Job drawing, mm, ordinate dimensions from the low corner. One solid piece. A direction names the side the tool comes from. Round coordinates to 2 decimals unless told otherwise and drop trailing zeros. Order: outer loops, then holes, each group sorted by start corner. A loop starts at its lowest first (then second) coordinate and runs counter-clockwise, first axis right, second up. Notation, with made-up numbers: (45.5, 78.5) -> (103.5, 78.5) arc R10 cw to (103.5, 96.5) -> close; hole circle Ø2 at (21.5, -22). An arc over 180 degrees is marked (long way). Return JSON: item names as keys, results as strings. Group by question number.
Q1. Which spindle directions (+Z, -Z, +X, -X, +Y, -Y) get a long thin tool onto all of the face, cutting with end or side? Do the marked faces 1, 2 and 3. Say none if no direction does.
Q2. Flat gauge pins, fed straight in: pin 1 (8 mm diameter, centred on y = 5.5, z = 30, fed in from -X); pin 2 (7.5 mm diameter, centred on x = 4.5, y = 6, fed in from +Z); pin 3 (3.5 mm diameter, centred on y = 7, z = 40, fed in from +X). Where does each tip first touch, or does it go through?
Q3. Cut at B-B (y = 11.75). Write the cut outline in (x, z).
Q4. Cut at C-C (x = 42.5). Write the cut outline in (y, z), then the cut area to 3 significant figures.
Q5. Mould opens along X. For the marked faces 4, 5 and 6 say: +X half, -X half, draft (parallel to the pull), parting line (faces both ways), or undercut.
Q6. Cut at A-A (z = 39). Write the cut outline in (x, y).
Q7. Probe line 1 along X through (y, z) = (5.5, 29); line 2 along X through (y, z) = (8, 40); line 3 along Z through (x, y) = (24, 6.5). List the from-to ranges inside material, lowest first.
Q8. Cut at D-D (z = 29). Write the cut outline in (x, y).
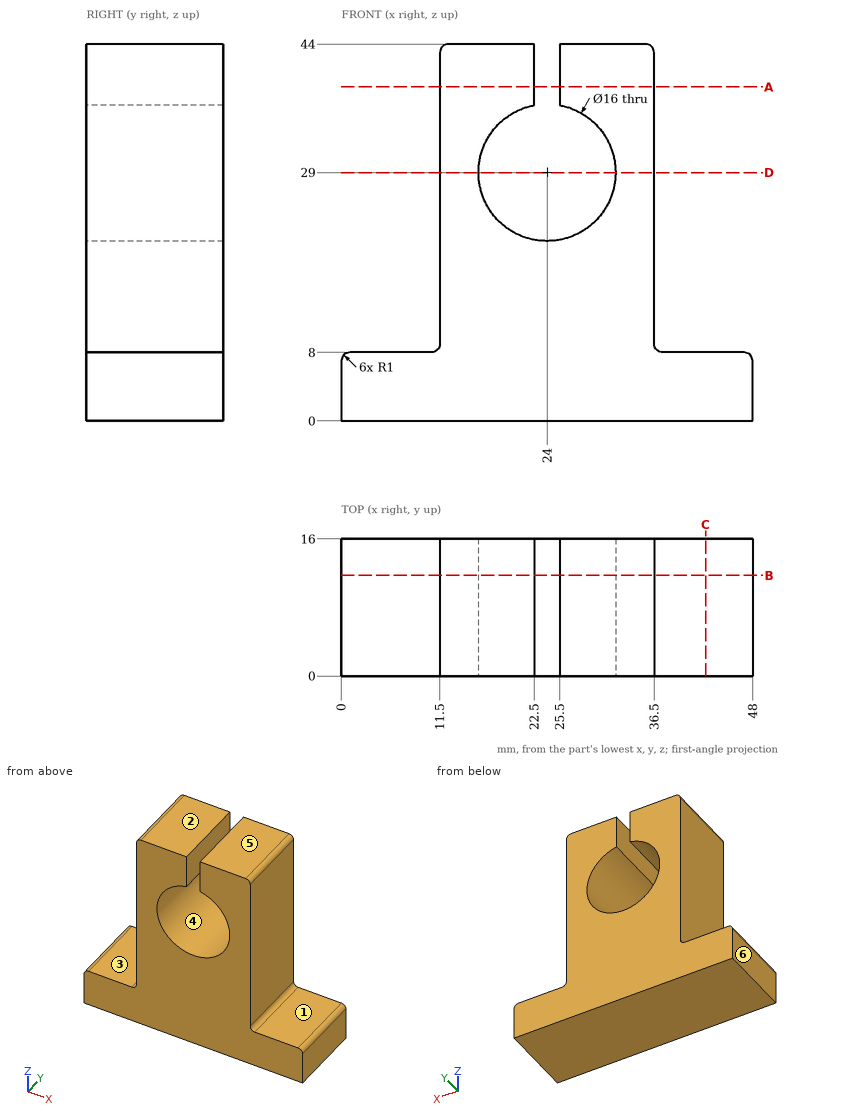
Solution:
{
 "1": {"face 1": "+Z, +X, +Y, -Y", "face 2": "+Z, +X, -X, +Y, -Y", "face 3": "+Z, -X, +Y, -Y"},
 "2": {"pin 1": "stops at x = 11.5", "pin 2": "stops at z = 8", "pin 3": "stops at x = 36.5"},
 "3": {"outline": "(0, 0) -> (48, 0) -> (48, 7) arc R1 ccw to (47, 8) -> (37.5, 8) arc R1 cw to (36.5, 9) -> (36.5, 43) arc R1 ccw to (35.5, 44) -> (25.5, 44) -> (25.5, 36.86) arc R8 cw (long way) to (22.5, 36.86) -> (22.5, 44) -> (12.5, 44) arc R1 ccw to (11.5, 43) -> (11.5, 9) arc R1 cw to (10.5, 8) -> (1, 8) arc R1 ccw to (0, 7) -> close"},
 "4": {"outline": "(0, 0) -> (16, 0) -> (16, 8) -> (0, 8) -> close", "area": "128 mm²"},
 "5": {"face 4": "undercut", "face 5": "draft", "face 6": "-X half"},
 "6": {"outline": "(11.5, 0) -> (22.5, 0) -> (22.5, 16) -> (11.5, 16) -> close; (25.5, 0) -> (36.5, 0) -> (36.5, 16) -> (25.5, 16) -> close"},
 "7": {"line 1": "x = 11.5 to 16, 32 to 36.5", "line 2": "x = 11.5 to 22.5, 25.5 to 36.5", "line 3": "z = 0 to 21"},
 "8": {"outline": "(11.5, 0) -> (16, 0) -> (16, 16) -> (11.5, 16) -> close; (32, 0) -> (36.5, 0) -> (36.5, 16) -> (32, 16) -> close"}
}
